Source: CAD feature listing. Evaluate the final solid. Frame: model axes, mm. Face numbers are marked on the shaded views. Round coordinates to 2 decimals unless told otherwise and drop trailing zeros. Order: outer loops, then holes, each group sorted by start corner. A loop starts at its lowest first (then second) coordinate and runs counter-clockwise, first axis right, second up. Notation, with made-up numbers: (19, -39) -> (32, -39) arc R19 ccw to (32, -28) -> close; hole circle Ø7 at (0, 40). An arc over 180 degrees is marked (long way). One line per item, written item: value. Start each with the question number.
1) Section D-D (z = -41.5). Return the cut outline in (x, y), and give its area (3 significant figures).
2) Section C-C (y = -5.5). Return the cut outline in (x, z).
3) Section B-B (x = -19.5). Return the cut outline in (y, z), and give its area (3 significant figures).
4) Mould query, pull axis Z, two halves, no side actions, for the marked faces 1, 2 and 3. Classes: pulls with the +Z half, pulls with the -Z half, needs draft (parallel to the pull), parting line crosses it, or undercut.
5) Ray query, L1, parallel to Y at x = -14, z = -46; L2, parallel to X at y = 5.5, z = 1; L3, parallel to Z at x = -5, y = 1.25. Return the intervals inside material, ascending.
6) Section A-A (z = 8.5). Return the cut outline in (x, y).
7) Pin query (flat end, axial travel): P1, Ø10, axis at x = 19.5, z = -45.5, coming from the -Y side; P2, Ø1.6, axis at x = 0, y = 7.5, coming from the -Z side; P3, Ø2, axis at x = 0.5, y = 6, coming from the +Z side. Return the tip coordinate at first contact, or that it passes through.
```python
from build123d import *

# Parameters (mm, degrees)
F0_W      = 50
F0_H      = 100
F1_DEPTH  = 2
F2_W      = 50
F2_H      = 2
F3_DEPTH  = 5
F4_W      = 10
F4_H      = 2
F5_DEPTH  = 15
F6_W      = 10
F6_H      = 2
F7_DEPTH  = 15
F8_W      = 20
F8_H      = 2
F9_DEPTH  = 10
F10_R     = 1.893356
F11_DEPTH = 3
F12_R     = 1.90716
F13_DEPTH = 3
F14_W     = 2
F14_H     = 20
F15_DEPTH = 10


with BuildPart() as f1:
    # F0 (on Front) → F1 (new body)
    with BuildSketch(Plane.XZ):
        Rectangle(F0_W, F0_H)
    extrude(amount=F1_DEPTH)

    # F2 (on face) → F3 (join)
    with BuildSketch(Plane(origin=(0, 0, 0), x_dir=(-1, 0, 0), z_dir=(0, 1, 0))):
        with Locations((0, -44)):
            Rectangle(F2_W, F2_H)
    extrude(amount=F3_DEPTH)

    # F4 (on face) → F5 (join)
    with BuildSketch(Plane(origin=(0, 0, -45), x_dir=(1, 0, 0), z_dir=(0, 0, -1))):
        with Locations((5, -4)):
            Rectangle(F4_W, F4_H)
    extrude(amount=F5_DEPTH)

    # F6 (on face) → F7 (join)
    with BuildSketch(Plane(origin=(0, 0, -45), x_dir=(1, 0, 0), z_dir=(0, 0, -1))):
        with Locations((-5, -4)):
            Rectangle(F6_W, F6_H)
    extrude(amount=F7_DEPTH)

    # F8 (on face) → F9 (join)
    with BuildSketch(Plane.XZ.offset(-3)):
        with Locations((0, -59)):
            Rectangle(F8_W, F8_H)
    extrude(amount=F9_DEPTH)

    # F10 (on face) → F11 (cut)
    with BuildSketch(Plane(origin=(0, 0, -60), x_dir=(1, 0, 0), z_dir=(0, 0, -1))):
        with Locations((-6.311274, 1.08402)):
            Circle(F10_R)
    extrude(amount=-F11_DEPTH, mode=Mode.SUBTRACT)

    # F12 (on face) → F13 (cut)
    with BuildSketch(Plane(origin=(0, 0, -60), x_dir=(1, 0, 0), z_dir=(0, 0, -1))):
        with Locations((6.244087, 0.790448)):
            Circle(F12_R)
    extrude(amount=-F13_DEPTH, mode=Mode.SUBTRACT)

    # F14 (on face) → F15 (join)
    with BuildSketch(Plane(origin=(0, 0, 0), x_dir=(-1, 0, 0), z_dir=(0, 1, 0))):
        Rectangle(F14_W, F14_H)
    extrude(amount=F15_DEPTH)


solid = f1.part
```
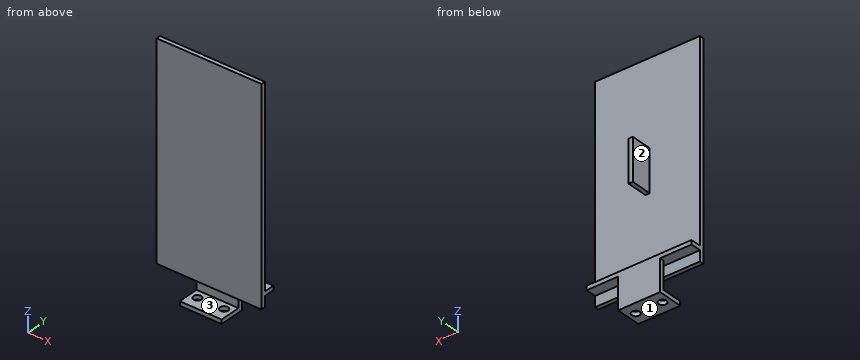
Findings:
1. outline: (-25, -2) -> (25, -2) -> (25, 0) -> (-25, 0) -> close
1. area: 100 mm2
2. outline: (-10, -60) -> (10, -60) -> (10, -58) -> (-10, -58) -> close
3. outline: (-2, -50) -> (0, -50) -> (0, -45) -> (5, -45) -> (5, -43) -> (0, -43) -> (0, 50) -> (-2, 50) -> close
3. area: 210 mm2
4. face 1: pulls with the -Z half
4. face 2: needs draft
4. face 3: undercut
5. L1: -2 to 0
5. L2: -1 to 1
5. L3: -60 to -58, -45 to -43
6. outline: (-25, -2) -> (25, -2) -> (25, 0) -> (1, 0) -> (1, 10) -> (-1, 10) -> (-1, 0) -> (-25, 0) -> close
7. P1: y = -2
7. P2: z = -10
7. P3: z = 10
